Build history of the part. All positions in model axes, mm. Coordinates: 2 decimals unless noted, no trailing zeros. Loops run counter-clockwise (first coordinate to the right, second up) from the corner with the lowest first, then second, coordinate; pieces in that order, holes last.
(1) Flat gauge pins, fed straight in: P1, Ø0.8, axis at x = -1, z = 14.5, coming from the -Y side; P2, Ø10, axis at x = -0.5, z = -2.5, coming from the +Y side; P3, Ø1.5, axis at x = 4, y = 1, coming from the -Z side. Where does each tip first touch, or does it go through?
(2) Slice it at C-C (z = -1.25). Give the cut face in (x, y), and give its area (3 significant figures).
(3) Slice it at A-A (x = 2.5). Give the cut face in (y, z), and give its area (3 significant figures).
(4) Wall check: L1, parallel to Z at x = 1.75, y = 1.4; L2, parallel to Y at x = 1.5, z = -11.25; L3, parallel to Z at x = -3.75, y = 2.9. Give the ranges that are in metal, low to high.
(5) Slice it at D-D (y = 3.65). Give the cut face in (x, z).
(6) Slice it at B-B (y = 0.45). Give the cut face in (x, z), and give its area (3 significant figures).
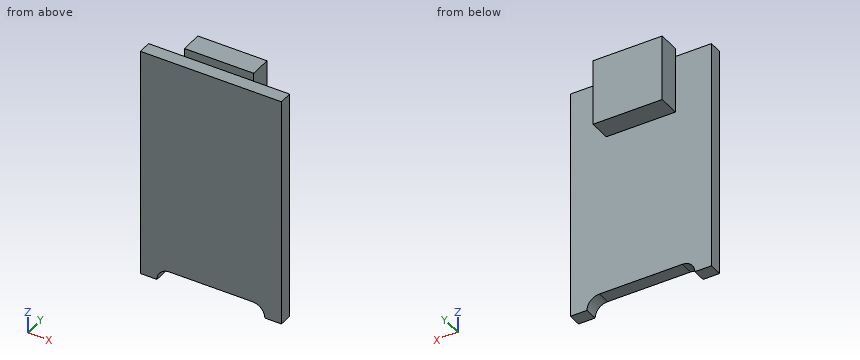
from build123d import *

# Parameters (mm, degrees)
SKETCH1_W           = 17
SKETCH1_H           = 28
BOSS_EXTRUDE1_DEPTH = 1.6
SKETCH2_W           = 8.34
SKETCH2_H           = 8
BOSS_EXTRUDE2_DEPTH = 2.6
CUT_EXTRUDE1_DEPTH  = 18.435882541


with BuildPart() as part:
    # Sketch1 → Boss-Extrude1 (new body)
    with BuildSketch(Plane(origin=(0, 0, 0), x_dir=(1, 0, 0), z_dir=(0, 1, 0))):
        Rectangle(SKETCH1_W, SKETCH1_H)
    extrude(amount=BOSS_EXTRUDE1_DEPTH)

    # Sketch2 → Boss-Extrude2 (add)
    with BuildSketch(Plane(origin=(0, 1.6, 0), x_dir=(1, 0, 0), z_dir=(0, 1, 0))):
        with Locations((0, -11)):
            Rectangle(SKETCH2_W, SKETCH2_H)
    extrude(amount=BOSS_EXTRUDE2_DEPTH)

    # Sketch3 → Cut-Extrude1 (cut, through all)
    with BuildSketch(Plane(origin=(0, 1.6, 0), x_dir=(1, 0, 0), z_dir=(0, 1, 0))):
        with BuildLine():
            Line((-5, 15.5), (5, 15.5))
            ThreePointArc((5, 15.5), (6.5, 14), (5, 12.5))
            Line((5, 12.5), (-5, 12.5))
            ThreePointArc((-5, 12.5), (-6.5, 14), (-5, 15.5))
        make_face()
    extrude(amount=-CUT_EXTRUDE1_DEPTH, mode=Mode.SUBTRACT)


solid = part.part
Response values:
1. P1: stops at y = 1.6
1. P2: stops at y = 1.6
1. P3: stops at z = -12.5
2. outline: (-8.5, 0) - (8.5, 0) - (8.5, 1.6) - (-8.5, 1.6) - close
2. area: 27.2 mm2
3. outline: (0, -12.5) - (1.6, -12.5) - (1.6, 7) - (4.2, 7) - (4.2, 15) - (1.6, 15) - (1.6, 14) - (0, 14) - close
3. area: 63.2 mm2
4. L1: z = -12.5 to 14
4. L2: y = 0 to 1.6
4. L3: z = 7 to 15
5. outline: (-4.17, 7) - (4.17, 7) - (4.17, 15) - (-4.17, 15) - close
6. outline: (-8.5, -14) - (-6.5, -14) arc R1.5 cw to (-5, -12.5) - (5, -12.5) arc R1.5 cw to (6.5, -14) - (8.5, -14) - (8.5, 14) - (-8.5, 14) - close
6. area: 457 mm2
